Geometry check sheet. Reference: the model listing, model coordinates, mm. Round coordinates to 2 decimals unless told otherwise and drop trailing zeros. Order: outer loops, then holes, each group sorted by start corner. A loop starts at its lowest first (then second) coordinate and runs counter-clockwise, first axis right, second up. Notation, with made-up numbers: (14, 21.25) - (28, 21.25) arc R34 cw to (28, 54.25) - close; hole circle Ø7 at (81.25, 58.25). An arc over 180 degrees is marked (long way). One line per question, with ' | ' between items. Start each with the question number.
Q1. Sectioned sample at B-B, the plane x = 42. Enter the section's corners in (y, z), then the cut area to 3 significant figures.
Q2. Sectioned sample at C-C, the plane z = 2.75. Enter the section's corners in (x, y), then the cut area to 3 significant figures.
Q3. Sectioned sample at D-D, the plane x = 18. Enter the section's corners in (y, z), then the cut area to 3 significant figures.
Q4. Material ranges on line 1 along Y through (x, z) = (33, 1.25); line 2 along Y through (x, z) = (54, 5.5); line 3 along X through (y, z) = (-11, 9.25) (3 decimals), recorded low to high.
Q5. Sectioned sample at A-A, the plane y = -52.5. Enter the section's corners in (x, z), then the cut area to 3 significant figures.
Q6. Mould release check, pull along X, two halves, no side actions. Record for faces 1 (the face through (54, -39, 10)), 2 (the face through (89.636, -49, 5)), 3 (the face through (2.487, -7.925, 4.93)), 4 (the face through (26.74, -66.75, 4.93)): +X half, -X half, draft (parallel to the pull), parting line (faces both ways), or undercut.
Autodesk Fusion 360 part; units mm, degrees
sketch "Sketch1" plane through (0, 0, 0) normal (0, 0, 1) x (1, 0, 0)
  line L0 (9.6355, -4.918) -> (79.6355, -4.918)
  line L1 (89.6355, -14.918) -> (89.6355, -84.918)
  line L2 (79.6355, -94.918) -> (-0.3645, -94.918)
  line L3 (-0.3645, -94.918) -> (-0.3645, -14.918)
  line L4 (-0.3645, -74.918) -> (19.6355, -94.918)
  circle A0 centre (39.6355, -54.918) radius 17.5
  arc A1 (9.6355, -4.918) -> (-0.3645, -14.918) centre (9.6355, -14.918) ccw
  arc A2 (89.6355, -14.918) -> (79.6355, -4.918) centre (79.6355, -14.918) ccw
  arc A3 (79.6355, -94.918) -> (89.6355, -84.918) centre (79.6355, -84.918) ccw
  point P0 (-0.3645, -4.918)
  point P1 (89.6355, -4.918)
  dimension "d1" = 90
  dimension "d2" = 90
  dimension "d3" = 20
  dimension "d4" = 20
  dimension "d5" = 35
  dimension "d6" = 40
  dimension "d7" = 40
  dimension "d8" = 10
  dimension "d9" = 10
  dimension "d10" = 10
extrude "Extrude1" add sketch "Sketch1" along normal blind 10 contours L0 L1 L2 L3 L4 A1 A2 A3
Determined:
1) outline: (-94.92, 0) - (-72.26, 0) - (-72.26, 10) - (-94.92, 10) - close; (-37.58, 0) - (-4.92, 0) - (-4.92, 10) - (-37.58, 10) - close | area: 553 mm2
2) outline: (-0.36, -74.92) - (19.64, -94.92) - (79.64, -94.92) arc R10 ccw to (89.64, -84.92) - (89.64, -14.92) arc R10 ccw to (79.64, -4.92) - (9.64, -4.92) arc R10 ccw to (-0.36, -14.92) - close; hole circle Ø35 at (39.64, -54.92) | area: 6,870 mm2
3) outline: (-93.28, 0) - (-4.92, 0) - (-4.92, 10) - (-93.28, 10) - close | area: 884 mm2
4) line 1: y = -94.92 to -71.11, -38.72 to -4.92 | line 2: y = -94.92 to -64.91, -44.92 to -4.92 | line 3: x = 0.435 to 88.836
5) outline: (-0.36, 0) - (22.3, 0) - (22.3, 10) - (-0.36, 10) - close; (56.97, 0) - (89.64, 0) - (89.64, 10) - (56.97, 10) - close | area: 553 mm2
6) face 1: draft | face 2: +X half | face 3: -X half | face 4: undercut
